from build123d import *

# Parameters (mm, degrees)
SKETCH3_W                    = 120
SKETCH3_H                    = 85
BASE_FLANGE1_DEPTH           = 6.35
EDGE_FLANGE1_STRIP_W         = 26.8732
EDGE_FLANGE1_STRIP_H         = 6.35
EDGE_FLANGE1_STRIP_CUT_DEPTH = 85
EDGE_FLANGE1_DEPTH           = 85
EDGE_FLANGE1_PROFILE_W       = 85
EDGE_FLANGE1_PROFILE_H       = 207.7009
EDGE_FLANGE1_PROFILE_R       = 7.9375
EDGE_FLANGE1_FLAT_DEPTH      = 6.35
FILLET1_R                    = 25


# Sheet-metal steps are written as plain solids
with BuildPart() as part:
    # Sketch3 → Base-Flange1 (new body)
    with BuildSketch(Plane(origin=(0, 0, 0), x_dir=(1, 0, 0), z_dir=(0, 1, 0))):
        Rectangle(SKETCH3_W, SKETCH3_H)
    extrude(amount=-BASE_FLANGE1_DEPTH)

    # Edge-Flange1 strip (across the edge) → Edge-Flange1 strip cut (cut)
    with BuildSketch(Plane(origin=(60, -6.35, -42.5), x_dir=(-1, 0, 0), z_dir=(0, 0, 1))):
        with Locations((-6.35, -3.175)):
            Rectangle(EDGE_FLANGE1_STRIP_W, EDGE_FLANGE1_STRIP_H)
    edge_flange1_strip_cut = extrude(amount=EDGE_FLANGE1_STRIP_CUT_DEPTH, mode=Mode.SUBTRACT)

    # Edge-Flange1 bend section (across the edge) → Edge-Flange1 (add)
    with BuildSketch(Plane(origin=(60, -6.35, -42.5), x_dir=(-1, 0, 0), z_dir=(0, 0, 1))):
        with BuildLine():
            Line((0, 0.7366), (6.35, 0.7366))
            ThreePointArc((6.35, 0.7366), (6.565745145, 0.215745145), (7.0866, 0))
            Line((7.0866, 0), (7.0866, -6.35))
            ThreePointArc((7.0866, -6.35), (2.075617084, -4.274382916), (0, 0.7366))
        make_face()
    edge_flange1 = extrude(amount=EDGE_FLANGE1_DEPTH)

    # Edge-Flange1 profile (on flange) → Edge-Flange1 flat (add)
    with BuildSketch(Plane(origin=(60, -6.35, 0), x_dir=(0, 0, -1), z_dir=(-1, 0, 0))):
        with Locations((0, 104.58705)):
            Rectangle(EDGE_FLANGE1_PROFILE_W, EDGE_FLANGE1_PROFILE_H)
        with Locations((0, 175.1)):
            Circle(EDGE_FLANGE1_PROFILE_R, mode=Mode.SUBTRACT)
    edge_flange1_flat = extrude(amount=EDGE_FLANGE1_FLAT_DEPTH)

    # Mirror1: Edge-Flange1 strip cut, Edge-Flange1, Edge-Flange1 flat across plane
    add(edge_flange1_strip_cut.mirror(Plane(origin=(0, 0, 0), x_dir=(0, 0, 1), z_dir=(1, 0, 0))), mode=Mode.SUBTRACT)
    add(edge_flange1.mirror(Plane(origin=(0, 0, 0), x_dir=(0, 0, 1), z_dir=(1, 0, 0))))
    add(edge_flange1_flat.mirror(Plane(origin=(0, 0, 0), x_dir=(0, 0, 1), z_dir=(1, 0, 0))))

    # Fillet1
    fillet1_edges = [part.edges().sort_by_distance(p)[0] for p in [
        (56.825, -214.7875, -42.5),
        (56.825, -214.7875, 42.5),
        (-56.825, -214.7875, 42.5),
        (-56.825, -214.7875, -42.5),
    ]]
    fillet(fillet1_edges, radius=FILLET1_R)


solid = part.part
Geometry: final body of the model. Coordinates: model frame, mm. A direction names the side the tool comes from. Give positions to 0.01 mm unless a question says otherwise; leave off trailing zeros. Write each loop counter-clockwise with the first axis right and the second up, starting at its lowest first coordinate (ties: lowest second). Pieces come first, ordered by that corner, then holes.
(1) Cut plane C-C, the plane z = -13. Return loops of the section in (x, y), then the cut area to 3 significant figures.
(2) Cut plane A-A, the plane y = -100. Return loops of the section in (x, z).
(3) Access query for faces 1 (the flat face through (-57, -214.788, 0)), 2 (the flat face through (-1, -6.35, -1)). Directions: +Z, -Z, +X, -X, +Y, -Y. A direction counts if a zero-diameter tool reaches every point of the face in a straight line with its end or side. Return the directions, or none.
(4) Cut plane B-B, the plane z = 0. Return loops of the section in (x, y), then the cut area to 3 significant figures.
(5) First-contact query: P1, Ø4, axis at x = -2.5, z = 26.5, coming from the -Y side. Flat tip, straight axial feed; report the tip coordinate or a pass-through.
(6) Mould query, pull axis X, two halves, no side actions, for faces 3 (the cylindrical face through (-56.87, -173.7, 1.72)), 4 (the flat face through (53.65, -112, 1)), 5 (the flat face through (60, -112, 1)). Classes: released by +X, released by -X, zero draft, split by the parting line, or undercut.
(7) Cut plane D-D, the plane y = -181.45. Return loops of the section in (x, z).
(8) Ray query, line 1 (X direction, y = -133.5, z = -35.5); line 2 (Y direction, x = -35, z = 28); line 3 (Y direction, x = -56, z = 0). Return the intervals inside material, ascending.
Values follow:
1. outline: (-60, -214.79) - (-53.65, -214.79) - (-53.65, -7.09) arc R0.74 cw to (-52.91, -6.35) - (52.91, -6.35) arc R0.74 cw to (53.65, -7.09) - (53.65, -214.79) - (60, -214.79) - (60, -7.09) arc R7.09 ccw to (52.91, 0) - (-52.91, 0) arc R7.09 ccw to (-60, -7.09) - close
1. area: 3,390 mm2
2. outline: (-60, -42.5) - (-53.65, -42.5) - (-53.65, 42.5) - (-60, 42.5) - close; (53.65, -42.5) - (60, -42.5) - (60, 42.5) - (53.65, 42.5) - close
3. face 1: +Z, -Z, +X, -X, -Y
3. face 2: +Z, -Z, -Y
4. outline: (-60, -214.79) - (-53.65, -214.79) - (-53.65, -189.39) - (-60, -189.39) - close; (-60, -173.51) - (-53.65, -173.51) - (-53.65, -7.09) arc R0.74 cw to (-52.91, -6.35) - (52.91, -6.35) arc R0.74 cw to (53.65, -7.09) - (53.65, -173.51) - (60, -173.51) - (60, -7.09) arc R7.09 ccw to (52.91, 0) - (-52.91, 0) arc R7.09 ccw to (-60, -7.09) - close; (53.65, -214.79) - (60, -214.79) - (60, -189.39) - (53.65, -189.39) - close
4. area: 3,190 mm2
5. P1: stops at y = -6.35
6. face 3: zero draft
6. face 4: undercut
6. face 5: released by +X
7. outline: (-60, -42.5) - (-53.65, -42.5) - (-53.65, -7.94) - (-60, -7.94) - close; (-60, 7.94) - (-53.65, 7.94) - (-53.65, 42.5) - (-60, 42.5) - close; (53.65, -42.5) - (60, -42.5) - (60, -7.94) - (53.65, -7.94) - close; (53.65, 7.94) - (60, 7.94) - (60, 42.5) - (53.65, 42.5) - close
8. line 1: x = -60 to -53.65, 53.65 to 60
8. line 2: y = -6.35 to 0
8. line 3: y = -214.79 to -189.39, -173.51 to -0.71
